from build123d import *

# Parameters (mm, degrees)
F0_W     = 81.99882
F0_H     = 10.50036
F1_DEPTH = 12
F2_T     = -1
F3_W     = 16.51
F3_H     = 11.00074
F4_DEPTH = 1
F5_W     = 70.61962
F5_H     = 6.92
F6_DEPTH = 2.54


with BuildPart() as f1:
    # F0 (on Front) → F1 (new body)
    with BuildSketch(Plane.XZ):
        Rectangle(F0_W, F0_H)
    extrude(amount=F1_DEPTH)

    # F2
    f2_openings = [f1.faces().sort_by_distance(p)[0] for p in [
        (0, -12, 0),
    ]]
    offset(amount=F2_T, openings=f2_openings)

    # F3 (on face) → F4 (cut)
    with BuildSketch(Plane(origin=(0, 0, -5.25018), x_dir=(1, 0, 0), z_dir=(0, 0, -1))):
        with Locations((-11.40841, 6.49963)):
            Rectangle(F3_W, F3_H)
    extrude(amount=-F4_DEPTH, mode=Mode.SUBTRACT)

    # F5 (on face) → F6 (cut)
    with BuildSketch(Plane.XY.offset(5.25018)):
        with Locations((0, -8.54)):
            Rectangle(F5_W, F5_H)
    extrude(amount=-F6_DEPTH, mode=Mode.SUBTRACT)


solid = f1.part
For this review, take the finished solid that the model builds, in its own axes (mm). A direction names the side the tool comes from. Round coordinates to 2 decimals unless told otherwise and drop trailing zeros. Write each loop counter-clockwise with the first axis right and the second up, starting at its lowest first coordinate (ties: lowest second). Pieces come first, ordered by that corner, then holes. Notation, with made-up numbers: (-26, -39) -> (-18, -39) arc R12 ccw to (-18, -25) -> close; hole circle Ø5 at (-26.75, -6). An arc over 180 degrees is marked (long way). Put each result on its own line as item: value.
Q1. Consider section B-B on z = 1.25. State the section outline as (x, y) points, and give its area (3 significant figures).
Determined:
outline: (-41, -12) -> (-40, -12) -> (-40, -1) -> (40, -1) -> (40, -12) -> (41, -12) -> (41, 0) -> (-41, 0) -> close
area: 104 mm^2
Q2. The part is to be moulded in two halves that separate along Z. For faces 1 (the flat face through (-1, -6, -5.25)), 2 (the flat face through (-1, -1, 0)), 3 (the flat face through (40.999, -6, 0)), say which applies: released by +Z, released by -Z, zero draft, split by the parting line, or undercut.
Determined:
face 1: released by -Z
face 2: undercut
face 3: zero draft
Q3. Machinability: for faces 4 (the flat face through (24, -12, -5)), 5 (the flat face through (-9, -4, 4.25)), which of the approach directions +Z, -Z, +X, -X, +Y, -Y give a long, thin tool a straight path to every point of the face, cutting with its end or side? Answer none if there is none.
Determined:
face 4: +Z, -Z, +X, -X, -Y
face 5: -Y
Q4. Clearance check with flat-ended pins moving along their axes: pin 1 Ø0.5 at (x, z) = (-7.5, -4.5) entering from -Y; pin 2 Ø5.5 at (x, y) = (23, -9) entering from +Z; pin 3 Ø4 at (x, z) = (29.5, 3.5) entering from +Y; pin 4 Ø0.8 at (x, z) = (15.5, 5) entering from -Y. State where each tip first meets the part, or that it passes through.
Determined:
pin 1: stops at y = -1
pin 2: stops at z = -4.25
pin 3: stops at y = 0
pin 4: stops at y = -5.08
Q5. To check wall thickness, follow L1, parallel to Z at x = 20, y = -1.5; L2, parallel to X at y = -3.5, z = 3.75; L3, parallel to Y at x = -6.5, z = 3.75. State the ranges of each line that lie inside material, in increasing order. Write a range as [from, to].
Determined:
L1: z = [-5.25, -4.25], [4.25, 5.25]
L2: x = [-41, -40], [40, 41]
L3: y = [-1, 0]
Q6. Consider section D-D on y = -3.5. State the section outline as (x, z) points.
Determined:
outline: (-41, -5.25) -> (-19.66, -5.25) -> (-19.66, -4.25) -> (-40, -4.25) -> (-40, 4.25) -> (40, 4.25) -> (40, -4.25) -> (-3.15, -4.25) -> (-3.15, -5.25) -> (41, -5.25) -> (41, 5.25) -> (-41, 5.25) -> close
Q7. Consider section A-A on y = -8.75. State the section outline as (x, z) points.
Determined:
outline: (-41, -5.25) -> (-19.66, -5.25) -> (-19.66, -4.25) -> (-40, -4.25) -> (-40, 4.25) -> (-35.31, 4.25) -> (-35.31, 5.25) -> (-41, 5.25) -> close; (-3.15, -5.25) -> (41, -5.25) -> (41, 5.25) -> (35.31, 5.25) -> (35.31, 4.25) -> (40, 4.25) -> (40, -4.25) -> (-3.15, -4.25) -> close
